```python
from build123d import *

# Parameters (mm, degrees)
SKETCH1_W          = 3.175
SKETCH1_H          = 36.83
BASE_DEPTH         = 3.175
SKETCH3_W          = 6.35
SKETCH3_H          = 5.715
RETAINER_DEPTH     = 3.175
TAB_DEPTH          = 3.175
FILLET1_R          = 1.27
FILLET2_R          = 2.54
CHAMFER1_SIZE      = 2.032
CUT_EXTRUDE1_REACH = 41.032


with BuildPart() as part:
    # Sketch1 → Base (new body)
    with BuildSketch(Plane.XY):
        Rectangle(SKETCH1_W, SKETCH1_H)
    extrude(amount=BASE_DEPTH)

    # Sketch3 → Retainer (add)
    with BuildSketch(Plane.ZY.offset(1.5875)):
        with Locations((6.35, 15.5575)):
            Rectangle(SKETCH3_W, SKETCH3_H)
        with Locations((6.35, -15.5575)):
            Rectangle(SKETCH3_W, SKETCH3_H)
    extrude(amount=-RETAINER_DEPTH)

    # Sketch5 → Tab (add)
    with BuildSketch(Plane.ZY.offset(1.5875)):
        Polygon((3.175, 9.525), (9.525, 9.525), (10.668, 10.16), (11.684, 10.16), (12.827, 9.525), (12.827, 7.62), (3.175, 7.62), align=None)
        Polygon((12.827, -7.62), (3.175, -7.62), (3.175, -9.525), (9.525, -9.525), (10.668, -10.16), (11.684, -10.16), (12.827, -9.525), align=None)
    extrude(amount=-TAB_DEPTH)

    # Fillet1
    fillet1_edges = [part.edges().sort_by_distance(p)[0] for p in [
        (0, 7.62, 3.175),
        (0, -7.62, 3.175),
    ]]
    fillet(fillet1_edges, radius=FILLET1_R)

    # Fillet2
    fillet2_edges = [part.edges().sort_by_distance(p)[0] for p in [
        (0, 18.415, 9.525),
        (0, -18.415, 9.525),
        (0, -18.415, 0),
        (0, 18.415, 0),
    ]]
    fillet(fillet2_edges, radius=FILLET2_R)

    # Chamfer1
    chamfer1_edges = [part.edges().sort_by_distance(p)[0] for p in [
        (0, 12.7, 9.525),
        (0, -12.7, 9.525),
    ]]
    chamfer(chamfer1_edges, length=CHAMFER1_SIZE)

    # Sketch6 → Cut-Extrude1 (cut, up to next)
    with BuildSketch(Plane(origin=(0, 18.415, 0), x_dir=(1, 0, 0), z_dir=(0, 1, 0)), mode=Mode.PRIVATE) as cut_extrude1_sk1:
        Polygon((-1.5875, -6.35), (-1.0795, -9.525), (-1.5875, -9.525), align=None)
    cut_extrude1_tool1 = extrude(cut_extrude1_sk1.sketch, amount=-CUT_EXTRUDE1_REACH, mode=Mode.PRIVATE) & part.part
    cut_extrude1 = cut_extrude1_tool1.solids().sort_by_distance((-1.418167, 18.415, 8.466667))[0]
    add(cut_extrude1, mode=Mode.SUBTRACT)

    # Mirror1: Cut-Extrude1 across plane
    add(cut_extrude1.mirror(Plane.ZX), mode=Mode.SUBTRACT)


solid = part.part
```
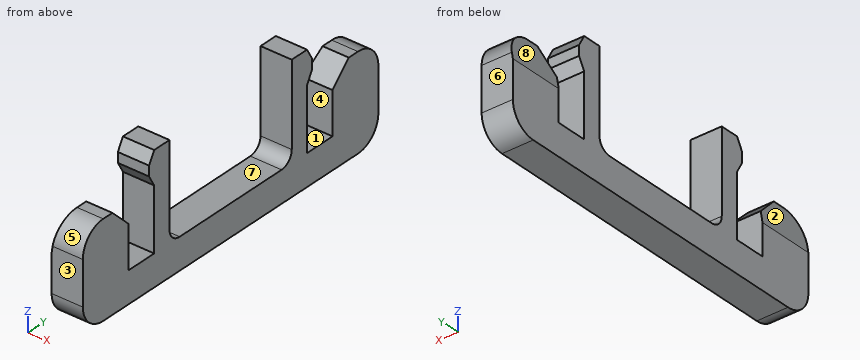
Read the model definition and answer for the solid it produces. Units are mm, in the model's axes. Face numbers are marked on the shaded views. A direction names the side the tool comes from. Give positions to 0.01 mm unless a question says otherwise; leave off trailing zeros. Loops run counter-clockwise (first coordinate to the right, second up) from the corner with the lowest first, then second, coordinate; pieces in that order, holes last.
Item 1: The part is cut by section A-A (z = 8). Write down the section's boundary in (x, y) (1 decimal).
Item 2: The part is cut by section B-B (z = 12). Write down the section's boundary in (x, y).
Item 3: Each of these flat-tipped pins is pushed along its axis until it touches: pin 1 Ø1.1 at (x, z) = (-0.5, 11) entering from +Y; pin 2 Ø1.6 at (x, y) = (0.5, -11) entering from +Z (3 decimals); pin 3 Ø0.6 at (x, y) = (-0.5, -15.5) entering from +Z (3 decimals); pin 4 Ø1 at (y, z) = (-10.5, 5) entering from +X. Where does it stop, or does it pass through?
Item 4: Find the intervals of material crossed by line 1 along Y through (x, z) = (-0.6, 4.75) (3 decimals); line 2 along Y through (x, z) = (1.1, 11.5); line 3 along Z through (x, y) = (-1.1, 1) (3 decimals), in increasing order.
Item 5: The mould has two halves that part along Y. Classify the marked faces 6, 7 and 8: released by +Y, released by -Y, zero draft, split by the parting line, or undercut.
Item 6: For the marked faces 1, 2, 3, 4 and 5, determine the directions among +Z, -Z, +X, -X, +Y, -Y from which every point of the face is accessible in a straight line to the end or side of a thin tool.
Taken from the geometry:
1. outline: (-1.6, -9.5) - (1.6, -9.5) - (1.6, -7.6) - (-1.6, -7.6) - close; (-1.6, 7.6) - (1.6, 7.6) - (1.6, 9.5) - (-1.6, 9.5) - close; (-1.3, -18.2) - (1.6, -18.2) - (1.6, -13.2) - (-1.3, -13.2) - close; (-1.3, 13.2) - (1.6, 13.2) - (1.6, 18.2) - (-1.3, 18.2) - close
2. outline: (-1.59, -9.98) - (1.59, -9.98) - (1.59, -7.62) - (-1.59, -7.62) - close; (-1.59, 7.62) - (1.59, 7.62) - (1.59, 9.98) - (-1.59, 9.98) - close
3. pin 1: stops at y = 10.16
3. pin 2: stops at z = 3.175
3. pin 3: stops at z = 9.525
3. pin 4: passes through
4. line 1: y = -18.415 to -12.7, -9.525 to -7.62, 7.62 to 9.525, 12.7 to 18.415
4. line 2: y = -10.16 to -7.62, 7.62 to 10.16
4. line 3: z = 0 to 3.175
5. face 6: released by +Y
5. face 7: undercut
5. face 8: zero draft
6. face 1: +X, -X
6. face 2: +Z, -X, -Y
6. face 3: +Z, -Z, +X, -X, -Y
6. face 4: +Z, +X, -X
6. face 5: +Z, +X, -X, -Y
